Input: dimensioned drawing with shaded views. Units: mm. Origin: part minimum x, y, z. A direction names the side the tool comes from. Round coordinates to 2 decimals unless told otherwise and drop trailing zeros. Loops run counter-clockwise (first coordinate to the right, second up) from the corner with the lowest first, then second, coordinate; pieces in that order, holes last.
1) Access query for the marked faces 1 and 2. Directions: +Z, -Z, +X, -X, +Y, -Y. A direction counts if a zero-diameter tool reaches every point of the face in a straight line with its end or side. Return the directions, or none.
2) Ray query, line 1 along Z through (x, y) = (20, 1); line 2 along Y through (x, z) = (22, 14). Return the intervals inside material, ascending.
3) Section B-B, the plane y = 24. Return loops of the section in (x, z), and give its area (3 significant figures).
4) Section C-C, the plane z = 3. Return loops of the section in (x, y) (3 decimals), and give its area (3 significant figures).
5) Section D-D, the plane y = 12. Return loops of the section in (x, z), and give its area (3 significant figures).
6) First-contact query: pin 1 (8 mm diameter, centred on y = 49.5, z = 56.5, fed in from +X); pin 2 (1.9 mm diameter, centred on y = 12, z = 31, fed in from -X); pin 3 (4 mm diameter, centred on x = 47.5, z = 9.5, fed in from +Y); pin 4 (1 mm diameter, centred on y = 53, z = 62, fed in from -X). Flat tips, straight axial feed; report the tip coordinate or a pass-through.
7) Section A-A, the plane z = 21. Return loops of the section in (x, y) (3 decimals), and give its area (3 significant figures).
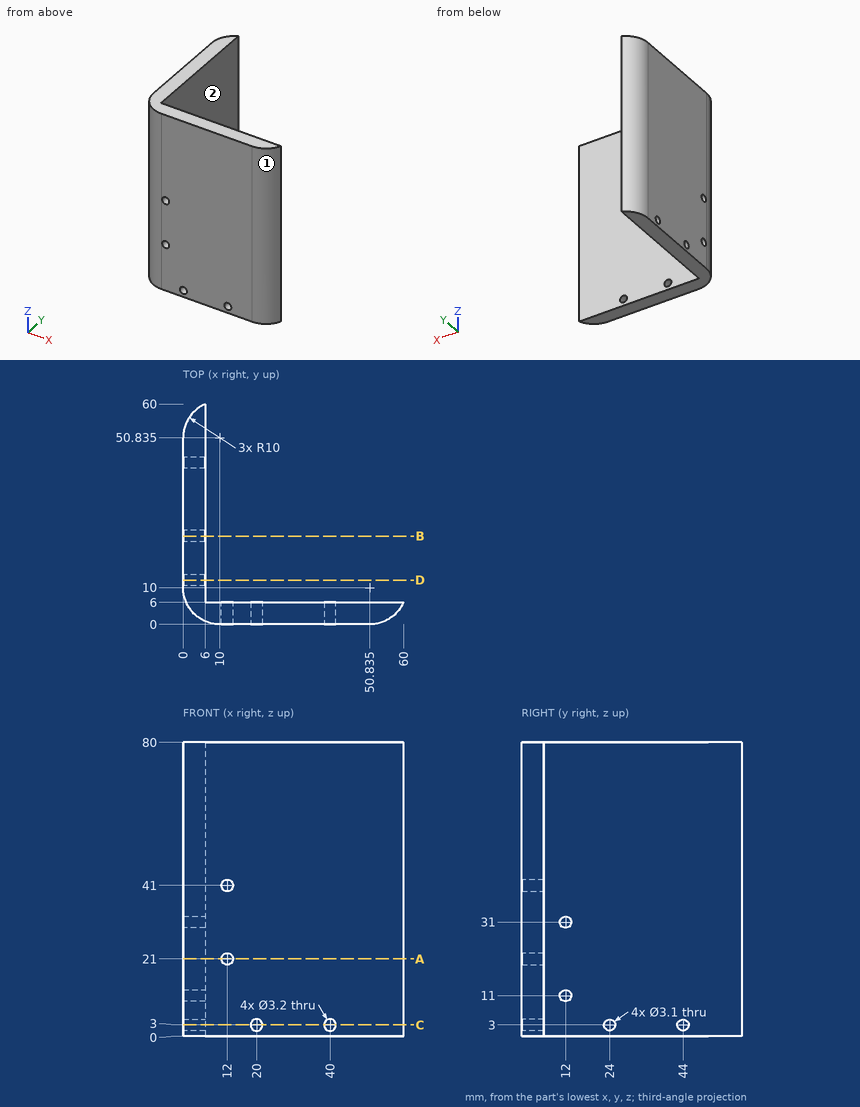
Final values:
1. face 1: +Z, -Z, +X, -Y
1. face 2: +Z, -Z, +X, +Y
2. line 1: z = 0 to 1.4, 4.6 to 80
2. line 2: y = 0 to 6
3. outline: (0, 0) - (6, 0) - (6, 1.45) - (0, 1.45) - close; (0, 4.55) - (6, 4.55) - (6, 80) - (0, 80) - close
3. area: 461 mm2
4. outline: (0, 10) arc R10 ccw to (10, 0) - (18.4, 0) - (18.4, 6) - (6, 6) - (6, 22.45) - (0, 22.45) - close; (0, 25.55) - (6, 25.55) - (6, 42.45) - (0, 42.45) - close; (0, 45.55) - (6, 45.55) - (6, 60) arc R10 ccw to (0, 50.835) - close; (21.6, 0) - (38.4, 0) - (38.4, 6) - (21.6, 6) - close; (41.6, 0) - (50.835, 0) arc R10 ccw to (60, 6) - (41.6, 6) - close
4. area: 556 mm2
5. outline: (0, 0) - (6, 0) - (6, 9.45) - (0, 9.45) - close; (0, 12.55) - (6, 12.55) - (6, 29.45) - (0, 29.45) - close; (0, 32.55) - (6, 32.55) - (6, 80) - (0, 80) - close
5. area: 443 mm2
6. pin 1: stops at x = 6
6. pin 2: passes through
6. pin 3: stops at y = 6
6. pin 4: stops at x = 0.14
7. outline: (0, 10) arc R10 ccw to (10, 0) - (10.4, 0) - (10.4, 6) - (6, 6) - (6, 60) arc R10 ccw to (0, 50.835) - close; (13.6, 0) - (50.835, 0) arc R10 ccw to (60, 6) - (13.6, 6) - close
7. area: 613 mm2
